CAD build for the part. Positions are in the model's coordinates, mm. A direction names the side the tool comes from. Give positions to 0.01 mm unless a question says otherwise; leave off trailing zeros. Loops run counter-clockwise (first coordinate to the right, second up) from the corner with the lowest first, then second, coordinate; pieces in that order, holes last.
Item 1: Which spindle directions (+Z, -Z, +X, -X, +Y, -Y) get a long thin tool onto all of the face, cutting with end or side? Do faces 5 (the cylindrical face through (9.654, -9.658, -11.976)), 6 (the flat face through (-43, -9, -6.35)), 7 (the cylindrical face through (16.331, -9.658, 2.282)). Say none if no direction does.
Item 2: Saw through at B-B on x = 0. Give the cut face in (y, z) (3 decimals), plus the area to 3 significant figures.
Item 3: Saw through at D-D on z = 1.5. Give the cut face in (x, y) (3 decimals), plus the area to 3 significant figures.
Item 4: Saw through at A-A on z = -9. Give the cut face in (x, y).
Item 5: Drop flat-ended pins along their axis: P1, Ø2, axis at y = -8, z = -4, coming from the -X side; P2, Ø9.5, axis at x = 36.5, y = -7.5, coming from the +Z side; P3, Ø5.5, axis at x = -52, y = -7.5, coming from the +Z side; P4, Ø2, axis at x = 48.5, z = -10, coming from the +Y side. Give the stop position or say it passes through.
Item 6: Probe probe 1 along X at (y, z) = (-12.5, -6.75); probe 2 along Y at (x, z) = (0, 1) (3 decimals); probe 3 along Z at (x, y) = (40, -10). List the from-to ranges inside material, lowest first.
Item 7: Mould opens along X. For faces 1 (the flat face through (43, -9, -6.35)), 2 (the cylindrical face through (8.2, -9.7, -0.8)), 3 (the cylindrical face through (-19.229, -9.658, -4.822)), 4 (the flat face through (8.89, -9, -6)) say: released by +X, released by -X, zero draft, split by the parting line, or undercut.
from build123d import *

# Parameters (mm, degrees)
F1_DEPTH = 19.05
F2_R     = 5.07999
F3_R     = 2.54
F4_DEPTH = 25.4
F5_R     = 2.54


# Not quite as in the source:
# - a fillet or chamfer is up to 0.001 mm smaller than in the source, because OpenCascade refuses the exact size


with BuildPart() as f1:
    # F0 (on Front) → F1 (new body)
    with BuildSketch(Plane.XZ):
        Polygon((17.78, -6.35), (17.78, 3.81), (-17.78, 3.81), (-17.78, -6.35), (-63.5, -6.35), (-63.5, -12.7), (-8.89, -12.7), (-8.89, 0), (8.89, 0), (8.89, -12.7), (63.5, -12.7), (63.5, -6.35), align=None)
    extrude(amount=F1_DEPTH)

    # F2 (radius 5.08 in the source; OpenCascade refuses exactly that, so slightly less here)
    f2_edges = [f1.edges().sort_by_distance(p)[0] for p in [
        (17.78, -9.525, 3.81),
        (17.78, -9.525, -6.35),
        (-17.78, -9.525, 3.81),
        (-17.78, -9.525, -6.35),
    ]]
    fillet(f2_edges, radius=F2_R)

    # F3 (on face) → F4 (cut)
    with BuildSketch(Plane.XY.offset(3.81)):
        with Locations((0, -9.525)):
            Circle(F3_R)
    extrude(amount=-F4_DEPTH, mode=Mode.SUBTRACT)

    # F5
    f5_edges = [f1.edges().sort_by_distance(p)[0] for p in [
        (8.89, -9.525, 0),
        (-8.89, -9.525, 0),
        (-8.89, -9.525, -12.7),
        (8.89, -9.525, -12.7),
    ]]
    fillet(f5_edges, radius=F5_R)


solid = f1.part
Results below:
1. face 5: -Z, +Y, -Y
1. face 6: +Z, -X, +Y, -Y
1. face 7: +Z, +X, +Y, -Y
2. outline: (-19.05, 0) - (-12.065, 0) - (-12.065, 3.81) - (-19.05, 3.81) - close; (-6.985, 0) - (0, 0) - (0, 3.81) - (-6.985, 3.81) - close
2. area: 53.2 mm2
3. outline: (-16.958, -19.05) - (16.958, -19.05) - (16.958, 0) - (-16.958, 0) - close; hole circle Ø5.08 at (0, -9.525)
3. area: 626 mm2
4. outline: (-63.5, -19.05) - (-8.89, -19.05) - (-8.89, 0) - (-63.5, 0) - close; (8.89, -19.05) - (63.5, -19.05) - (63.5, 0) - (8.89, 0) - close
5. P1: stops at x = -19.41
5. P2: stops at z = -6.35
5. P3: stops at z = -6.35
5. P4: stops at y = 0
6. probe 1: x = -63.5 to -8.89, 8.89 to 63.5
6. probe 2: y = -19.05 to -12.065, -6.985 to 0
6. probe 3: z = -12.7 to -6.35
7. face 1: zero draft
7. face 2: undercut
7. face 3: released by -X
7. face 4: undercut
